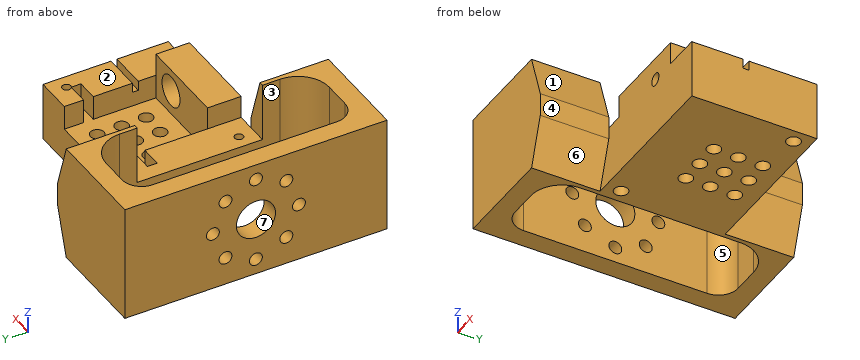
Autodesk Inventor part; units mm, degrees
ref_plane "YZ Plane" through (0, 0, 0) normal (1, 0, 0) x (0, 1, 0)
ref_plane "XZ Plane" through (0, 0, 0) normal (0, 1, 0) x (-1, 0, 0)
ref_plane "XY Plane" through (0, 0, 0) normal (0, 0, 1) x (1, 0, 0)
sketch "Sketch2" plane through (0, 0, 0) normal (0, 0, 1) x (1, 0, 0)
  line L0 (0, 0) -> (42, 0)
  line L1 (42, 0) -> (42, 32)
  line L2 (42, 32) -> (0, 32)
  line L3 (0, 32) -> (0, 0)
  dimension "d0" = 42
  dimension "d1" = 32
extrude "Body_body" add sketch "Sketch2" along normal blind 15
sketch "Sketch4" plane through (0, 0, 15) normal (0, 0, 1) x (1, 0, 0)
  line L0 (42, 32) -> (0, 32)
  line L1 (0, 32) -> (0, 0)
  line L2 (4, 24.6) -> (9.5, 24.6)
  line L3 (9.5, 24.6) -> (9.5, 8.6)
  line L4 (9.5, 8.6) -> (32.5, 8.6)
  line L5 (32.5, 8.6) -> (32.5, 24.6)
  line L6 (32.5, 24.6) -> (38, 24.6)
  line L7 (42, 0) -> (42, 32)
  line L8 (0, 0) -> (42, 0)
  line L9 (4, 24.6) -> (4, 27.1)
  line L10 (4, 27.1) -> (9.5, 27.1)
  line L11 (9.5, 27.1) -> (9.5, 32)
  line L12 (38, 27.1) -> (38, 24.6)
  line L13 (38, 27.1) -> (32.5, 27.1)
  line L14 (32.5, 27.1) -> (32.5, 32)
  line L15 (9.5, 32) -> (32.5, 32)
  line L16 (21, 36.5125) -> (21, -47.625) construction
  point P0 (4.9935, 32)
  point P1 (37, 32)
  dimension "d6" = 5.5
  dimension "d7" = 16
  dimension "d8" = 23
  dimension "d11" = 8.6
  dimension "d14" = 2.5
  dimension "d15" = 2.5
  dimension "d22" = 42
  dimension "d23" = 21
  dimension "d24" = 23
  dimension "d25" = 11.5
  dimension "d26" = 4.9
  dimension "d27" = 4.9
  dimension "d28" = 5.5
extrude "Servo_Intake" cut sketch "Sketch4" against normal blind 6.25 contours L14 L13 L12 L6 L5 L4 L3 L2 L9 L10 L11 L0
sketch "Sketch5" plane through (0, 0, 15) normal (0, 0, 1) x (1, 0, 0)
  line L0 (42, 0) -> (42, 32)
  line L1 (42, 14.6) -> (42, 13.1)
  line L2 (-29.647, 13.85) -> (54.8226, 13.85) construction
  line L3 (0, 0) -> (42, 0)
  line L4 (32.5, 8.6) -> (9.5, 8.6)
  line L5 (42, 13.1) -> (32.5, 13.1)
  line L6 (32.5, 13.1) -> (32.5, 14.6)
  line L7 (32.5, 24.6) -> (32.5, 8.6)
  line L8 (42, 14.6) -> (32.5, 14.6)
  dimension "d171" = 1.5
  dimension "d211" = 4.5
extrude "Cable_Opening" cut sketch "Sketch5" against normal blind 2.5
sketch "Sketch6" plane through (0, 0, 15) normal (0, 0, 1) x (1, 0, 0)
  circle A0 centre (3.5, 28) radius 1.1 construction
  circle A1 centre (38.5, 28) radius 1.1
  circle A2 centre (38.5, 4) radius 1.1 construction
  circle A3 centre (3.5, 4) radius 1.1
  line L0 (21, 34.35) -> (21, -13.275) construction
  line L1 (-20.6375, 16) -> (66.675, 16) construction
  line L2 (42, 14.6) -> (42, 32)
  line L3 (0, 32) -> (0, 0)
  line L4 (9.5, 32) -> (0, 32)
  line L5 (0, 0) -> (42, 0)
  point P0 (42, 12.35)
  point P1 (0, 12.35)
  dimension "d29" = 2.2
  dimension "d30" = 2.2
  dimension "d31" = 2.2
  dimension "d32" = 2.2
  dimension "d33" = 42
  dimension "d34" = 21
  dimension "d35" = 32
  dimension "d36" = 16
  dimension "d37" = 35
  dimension "d38" = 17.5
  dimension "d39" = 24
  dimension "d40" = 12
extrude "Holes_Mounting_Screws" cut sketch "Sketch6" against normal up to surface (15 mm away)
sketch "Sketch10" plane through (0, 0, 15) normal (0, 0, 1) x (1, 0, 0)
  line L0 (32.5, 8.6) -> (9.5, 8.6)
  line L1 (9.5, 8.6) -> (32.5, 8.6)
  line L2 (32.5, 8.6) -> (32.5, 0)
  line L3 (32.5, 0) -> (9.5, 0)
  line L4 (9.5, 0) -> (9.5, 8.6)
  line L5 (9.5, 8.6) -> (9.5, 24.6)
  line L6 (32.5, 24.6) -> (32.5, 14.6)
  point P0 (0, 0)
  point P1 (9.5, 12.35)
  point P2 (32.5, 12.35)
extrude "Socket" add sketch "Sketch10" along normal blind 5.8
sketch "Sketch11" plane through (9.5, 8.6, 8.75) normal (0, 1, 0) x (1, 0, 0)
  circle A0 centre (16.25, -6.25) radius 1.6
  line L0 (-9.5, -6.05) -> (-9.5, -3.55)
  line L1 (32.5, 8.75) -> (32.5, -6.25)
  point P0 (-9.5, 8.75)
  point P1 (0, -6.25)
  dimension "d65" = 3.2
  dimension "d69" = 16.25
extrude "Shaft_Opening" cut sketch "Sketch11" against normal up to surface (8.6 mm away)
sketch "Sketch12" plane through (9.5, 8.6, 8.75) normal (0, 1, 0) x (1, 0, 0)
  circle A0 centre (16.25, -6.25) radius 4
  circle A1 centre (16.25, -6.25) radius 1.6
  point P0 (-9.5, 8.75)
  dimension "d73" = 8
extrude "Shaft_Pocket" cut sketch "Sketch12" against normal blind 5.7
sketch "Sketch15" plane through (0, 0, 15) normal (0, 0, 1) x (1, 0, 0)
  line L0 (9.5, 32) -> (0, 32)
  line L1 (0, 0) -> (9.5, 0)
  line L2 (42, 32) -> (32.5, 32)
  line L3 (32.5, 0) -> (42, 0)
  line L4 (42, 32) -> (0, 32)
  line L5 (0, 32) -> (0, 44.5)
  line L6 (0, 44.5) -> (-20, 44.5)
  line L7 (0, 32) -> (5, 32)
  line L8 (5, 32) -> (5, 49.5)
  line L9 (5, 49.5) -> (-25, 49.5)
  line L10 (0, 0) -> (0, -12.5)
  line L11 (0, -12.5) -> (-20, -12.5)
  line L12 (-20, -12.5) -> (-20, 44.5)
  line L13 (0, 0) -> (5, 0)
  line L14 (5, 0) -> (5, -17.5)
  line L15 (5, -17.5) -> (-25, -17.5)
  line L16 (-25, -17.5) -> (-25, 49.5)
  line L17 (0, 32) -> (0, 0)
  dimension "d111" = 12.5
  dimension "d113" = 5
  dimension "d114" = 17.5
  dimension "d116" = 12.5
  dimension "d118" = 5
  dimension "d119" = 17.5
  dimension "d120" = 30
  dimension "d161" = 5
  dimension "d175" = 30
  dimension "d191" = 5
  dimension "d212" = 25
extrude "Connection_Adapter" add sketch "Sketch15" along normal mid plane 30 contours L0 L5 L6 L12 L11 L10 L1 L14 L15 L16 L9 L8
sketch "Sketch17" plane through (-20, -12.5, 30) normal (1, 0, 0) x (0, 0, -1)
  circle A0 centre (15, 28.5) radius 11 construction
  line L0 (30, 57) -> (0, 57)
  line L1 (30, 0) -> (0, 0)
  line L2 (0, 0) -> (0, 57)
  line L3 (30, 57) -> (30, 0)
  line L4 (15, 15.142) -> (15, 40.542) construction
  line L5 (1.1452, 28.5) -> (27.1241, 28.5) construction
  line L6 (4.9901, 18.4901) -> (35.9566, 49.4566) construction
  line L7 (5.2574, 38.2426) -> (22.7782, 20.7218) construction
  circle A1 centre (7.2218, 20.7218) radius 1.65
  circle A2 centre (4, 28.5) radius 1.65
  circle A3 centre (7.2218, 36.2782) radius 1.65
  circle A4 centre (15, 39.5) radius 1.65
  circle A5 centre (15, 17.5) radius 1.65
  circle A6 centre (22.7782, 20.7218) radius 1.65
  circle A7 centre (26, 28.5) radius 1.65
  circle A8 centre (22.7782, 36.2782) radius 1.65
  point P0 (30, 12.5)
  dimension "d121" = 22
  dimension "d122" = 57
  dimension "d123" = 28.5
  dimension "d124" = 30
  dimension "d125" = 15
  dimension "d126" = 3.3
  dimension "d127" = 3.3
  dimension "d128" = 3.3
  dimension "d129" = 3.3
  dimension "d130" = 3.3
  dimension "d131" = 3.3
  dimension "d132" = 3.3
  dimension "d133" = 3.3
  dimension "d134" = 45
  dimension "d135" = 45
extrude "Connector_Holes" cut sketch "Sketch17" against normal up to surface (5 mm away) contours A1 | A2 | A3 | A4 | A5 | A6 | A7 | A8
sketch "Sketch19" plane through (-20, -12.5, 30) normal (1, 0, 0) x (0, 0, -1)
  circle A0 centre (15, 28.5) radius 5
  line L0 (30, 0) -> (0, 0)
  line L1 (30, 57) -> (0, 57)
  line L2 (30, 57) -> (30, 0)
  line L3 (0, 0) -> (0, 57)
  point P0 (30, 12.5)
  dimension "d140" = 10
  dimension "d141" = 57
  dimension "d142" = 28.5
  dimension "d143" = 30
  dimension "d144" = 15
extrude "Connector_Center_Hole" cut sketch "Sketch19" against normal up to surface (5 mm away) contours A0
sketch "Sketch22" plane through (0, 0, 0) normal (0, 0, -1) x (-1, 0, 0)
  circle A0 centre (-38.5, 28) radius 1.1
  line L0 (-3.5, 36.8375) -> (-3.5, -9.2) construction
  line L1 (-42, 0) -> (-42, 32)
  line L2 (0, -12.5) -> (0, 44.5)
  line L3 (-5, 0) -> (-42, 0)
  line L4 (-42, 32) -> (-5, 32)
  circle A1 centre (-3.5, 4) radius 1.75
  circle A2 centre (-38.5, 28) radius 1.75
  circle A3 centre (-3.5, 4) radius 1.1
  circle A4 centre (-38.5, 28) radius 1.1
  point P0 (0, 0)
  point P1 (0, -1)
  dimension "d167" = 3.5
  dimension "d168" = 3.5
  dimension "d176" = 2.25
  dimension "d177" = 1.75
extrude "Pocket_Inserts" cut sketch "Sketch22" against normal blind 5
fillet "Fillet4" radius 8 2 edges at (0, 44.5, 15) (0, -12.5, 15)
chamfer "Chamfer1" distance 12 angle 18 1 edges at (5, -8.75, 30) measured on face at (5, -11.6667, 15)
chamfer "Chamfer2" distance 12 angle 18 1 edges at (5, -8.75, 0) measured on face at (5, -11.6667, 11)
chamfer "Chamfer3" distance 12 angle 18 1 edges at (5, 40.75, 30) measured on face at (5, 43.6667, 15)
chamfer "Chamfer4" distance 12 angle 18 1 edges at (5, 40.75, 0) measured on face at (5, 43.6667, 11)
fillet "Fillet5" radius 5 2 edges at (-20, -12.5, 15) (-20, 44.5, 15)
sketch "Sketch24" plane through (0, 0, 8.75) normal (0, 0, 1) x (1, 0, 0)
  circle A0 centre (14.75, 26.6) radius 1.75
  line L0 (9.5, 32) -> (32.5, 32)
  line L1 (9.5, 27.1) -> (9.5, 32)
  line L2 (32.5, 32) -> (32.5, 27.1)
  point P0 (0, 0)
  dimension "d192" = 3.5
  dimension "d193" = 5.4
  dimension "d194" = 5.25
  dimension "d200" = 23
extrude "Heat_dissipation_Hole" cut sketch "Sketch24" against normal up to surface (8.75 mm away)
pattern_linear "Rectangular Pattern1" count 3 spacing 6.25 along (1, 0, 0) count 3 spacing 6.25 along (0, -1, 0) of "Heat_dissipation_Hole"
equation "\"d15\" = d14"
equation "\"d23\" = 0.5 * d22"
equation "\"d25\" = 0.5 * d24"
equation "\"d27\" = d26"
equation "\"d28\" = d6"
equation "\"d34\" = 0.5 * d33"
equation "\"d36\" = 0.5 * d35"
equation "\"d38\" = 0.5 * d37"
equation "\"d40\" = 0.5 * d39"
equation "\"d65\" = d70"
equation "\"d142\" = 0.5 * d141"
equation "\"d144\" = 0.5 * d143"
equation "\"d167\" = d168"
properties part number "EDMO1-0_Body" material "PLA"
Design review of the part built by this model. Coordinates are the model's own, in mm. Face numbers are marked on the shaded views. A direction names the side the tool comes from. Round coordinates to 2 decimals unless told otherwise and drop trailing zeros. Order: outer loops, then holes, each group sorted by start corner. A loop starts at its lowest first (then second) coordinate and runs counter-clockwise, first axis right, second up. Notation, with made-up numbers: (19, 89.25) - (68, 89.25) arc R16 cw to (68, 108.25) - close; hole circle Ø7 at (-7, 53). An arc over 180 degrees is marked (long way). Return JSON: item names as keys, results as strings.
Q1. Wall thickness on L1, parallel to Y at x = 21, z = 2; L2, parallel to X at y = 28, z = 10.75; L3, parallel to Z at x = 25.75, y = 2.15: over which ranges is each line inside the solid? List them lowest first. Write a range as [from, to].
Computed values:
{"L1": "y = [0, 12.35], [15.85, 18.6], [22.1, 24.85], [28.35, 32]", "L2": "x = [-25, -20], [0, 9.5], [32.5, 37.4], [39.6, 42]", "L3": "z = [0, 13.4], [16.6, 20.8]"}
Q2. For pin 1 Ø6 at (x, y) = (14.5, 19) entering from -Z; pin 2 Ø1.2 at (x, z) = (38, 13.5) entering from +Y; pin 3 Ø4.5 at (x, y) = (14.75, 26.6) entering from +Z; pin 4 Ø1.2 at (x, z) = (35.5, 14) entering from -Y, all flat-tipped, find the tip position at first contact; note any pin that passes through.
Computed values:
{"pin 1": "stops at z = 0", "pin 2": "stops at y = 32", "pin 3": "stops at z = 8.75", "pin 4": "stops at y = 0"}
Q3. Consider section C-C on x = -17.5. Write out the cut boundary in (y, z).
Computed values:
{"outline": "(-17.5, 0) - (-11.83, 0) - (-11.83, 30) - (-17.5, 30) - close; (43.83, 0) - (49.5, 0) - (49.5, 30) - (43.83, 30) - close"}
Q4. Consider section B-B on z = 26. Write out the cut boundary in (x, y).
Computed values:
{"outline": "(-25, -17.5) - (2.4, -17.5) - (2.4, 0) - (0, 0) - (0, -4.5) arc R8 cw to (-8, -12.5) - (-15, -12.5) arc R5 cw to (-20, -7.5) - (-20, 14.35) - (-25, 14.35) - close; (-25, 17.65) - (-20, 17.65) - (-20, 39.5) arc R5 cw to (-15, 44.5) - (-8, 44.5) arc R8 cw to (0, 36.5) - (0, 32) - (2.4, 32) - (2.4, 49.5) - (-25, 49.5) - close"}
Q5. Consider section A-A on y = -1.5. Write out the cut boundary in (x, z).
Computed values:
{"outline": "(-25, 0) - (-20, 0) - (-20, 30) - (-25, 30) - close; (0, 0) - (1.1, 0) - (5, 12) - (5, 18) - (1.1, 30) - (0, 30) - close"}
Q6. Machinability: for the marked faces 4, 5, 6 and 7, which of the approach directions +Z, -Z, +X, -X, +Y, -Y give a long, thin tool a straight path to every point of the face, cutting with its end or side? Answer none if there is none.
Computed values:
{"face 4": "+Z, -Z, +X, -Y", "face 5": "+Z, -Z", "face 6": "-Z, +X, -Y", "face 7": "-X"}
Q7. The part is to be moulded in two halves that separate along X. For the marked faces 1, 2 and 3, say which applies: pulls with the +X half, pulls with the -X half, needs draft (parallel to the pull), parting line crosses it, or undercut.
Computed values:
{"face 1": "pulls with the +X half", "face 2": "needs draft", "face 3": "undercut"}
